Can you work these out from the model? Positions are in its coordinate system, mm. A direction names the side the tool comes from. Round coordinates to 2 decimals unless told otherwise and drop trailing zeros. Write each loop counter-clockwise with the first axis right and the second up, starting at its lowest first coordinate (ties: lowest second). Pieces come first, ordered by that corner, then holes. Notation, with made-up numbers: (-35, 58.5) - (-7, 58.5) arc R7 ccw to (-7, 66.5) - close; hole circle Ø8 at (-23.75, 83.25). An arc over 180 degrees is marked (long way). One line per item, written item: value. Start each with the question number.
(1) I'm going to push flat-ended pins straight in: pin 1 Ø5 at (x, z) = (25.5, 40.5) entering from +Y; pin 2 Ø2 at (x, y) = (36, -7.5) entering from -Z; pin 3 Ø12 at (y, z) = (29, 31.5) entering from +X. Where does each tip first touch, or does it pass through?
(2) I want a section at B-B on x = -19. List the corners of the cut face in (y, z) for me.
(3) If I drill on L1, parallel to X at y = -10, z = 30; L2, parallel to Y at x = 8, z = 18.5; L3, parallel to X at y = -7.85, z = 30, over which ranges is the centre line in solid material (lowest first)? Write a range as from..to.
(4) I want a section at D-D on z = 24. Give the number of separate pieces and of enclosed holes in the cut face, plus the area to 3 significant figures.
(5) I want a section at A-A on y = 18.4. List the corners of the cut face in (x, z) for me, plus the area to 3 significant figures.
(6) I want a section at C-C on y = -7.5. List the corners of the cut face in (x, z) for me.
(7) Thinking about a two-plate mould opening in X: for faces 4 (the face through (9.513, -5.748, 29.58)), 5 (the face through (-4.079, -5.593, 29.58)), 6 (the face through (9.506, 3, 30)), 7 (the face through (-27, -5.6, 20)), which applies, +X half, -X half, draft (parallel to the pull), parting line (faces both ways), or undercut?
(8) On a 3-axis mill with a long thin cutter (end or side, diameter ignored), from which of +Z, -Z, +X, -X, +Y, -Y can I reach the whole of each face in a straight line? I mean faces 1 (the face through (7.985, 8.056, 43.491)), 2 (the face through (-1.228, 35, 30)), 3 (the face through (27, -5.6, 20)). Say none if no direction works.
from build123d import *

# Parameters (mm, degrees)
BOSS_EXTRUDE1_DEPTH      = 60
SKETCH2_R                = 12
SKETCH2_R_2              = 10
BOSS_EXTRUDE3_DEPTH      = 3
SKETCH10_R               = 10
CUT_EXTRUDE3_DEPTH       = 53
SKETCH11_5_R             = 15
CUT_EXTRUDE4_DEPTH       = 23
SKETCH11_R               = 17
SKETCH11_R_2             = 15
BOSS_EXTRUDE7_DEPTH      = 3
BOSS_EXTRUDE7_DEPTH_BACK = 3


with BuildPart() as part:
    # Sketch1 → Boss-Extrude1 (new body)
    with BuildSketch(Plane.XY):
        with BuildLine():
            Line((-47.49441662, -13.6), (52.50558338, -13.6))
            Line((52.50558338, -13.6), (52.50558338, -8.6))
            Line((52.50558338, -8.6), (16.50558338, -8.6))
            ThreePointArc((16.50558338, -8.6), (9.434515568, -5.671067812), (6.50558338, 1.4))
            Line((6.50558338, 1.4), (6.50558338, 41.4))
            Line((6.50558338, 41.4), (-1.227749954, 41.4))
            Line((-1.227749954, 41.4), (-1.227749954, 1.4))
            ThreePointArc((-1.227749954, 1.4), (-4.156682142, -5.671067812), (-11.227749954, -8.6))
            Line((-11.227749954, -8.6), (-47.49441662, -8.6))
            Line((-47.49441662, -8.6), (-47.49441662, -13.6))
        make_face()
    extrude(amount=BOSS_EXTRUDE1_DEPTH)

    # Sketch2 → Boss-Extrude3 (add)
    with BuildSketch(Plane(origin=(0, -8.6, 0), x_dir=(1, 0, 0), z_dir=(0, 1, 0))):
        with Locations((-24.49441662, -30)):
            Circle(SKETCH2_R)
        with Locations((-24.49441662, -30)):
            Circle(SKETCH2_R_2, mode=Mode.SUBTRACT)
        with Locations((29.50558338, -30)):
            Circle(SKETCH2_R)
        with Locations((29.50558338, -30)):
            Circle(SKETCH2_R_2, mode=Mode.SUBTRACT)
    extrude(amount=BOSS_EXTRUDE3_DEPTH)

    # Sketch10 → Cut-Extrude3 (cut)
    with BuildSketch(Plane(origin=(0, -8.6, 0), x_dir=(1, 0, 0), z_dir=(0, 1, 0))):
        with Locations((-24.49441662, -30)):
            Circle(SKETCH10_R)
        with Locations((29.50558338, -30)):
            Circle(SKETCH10_R)
    extrude(amount=-CUT_EXTRUDE3_DEPTH, mode=Mode.SUBTRACT)

    # Sketch11_5 → Cut-Extrude4 (cut)
    with BuildSketch(Plane(origin=(6.50558338, 0, 0), x_dir=(0, 0, -1), z_dir=(1, 0, 0))):
        with Locations((-30, 18.4)):
            Circle(SKETCH11_5_R)
        with BuildLine():
            Line((-60, 41.4), (-60, 31.869694824))
            ThreePointArc((-60, 31.869694824), (-57.186392619, 38.586392619), (-50.469694824, 41.4))
            Line((-50.469694824, 41.4), (-60, 41.4))
        make_face()
        with BuildLine():
            Line((0, 41.4), (-9.606995457, 41.4))
            ThreePointArc((-9.606995457, 41.4), (-3.020943995, 38.379056005), (0, 31.793004543))
            Line((0, 31.793004543), (0, 41.4))
        make_face()
    extrude(amount=-CUT_EXTRUDE4_DEPTH, mode=Mode.SUBTRACT)

    # Sketch11 → Boss-Extrude7 (add, two sides)
    with BuildSketch(Plane(origin=(6.50558338, 0, 0), x_dir=(0, 0, -1), z_dir=(1, 0, 0))) as boss_extrude7_sk:
        with Locations((-30, 18.4)):
            Circle(SKETCH11_R)
        with Locations((-30, 18.4)):
            Circle(SKETCH11_R_2, mode=Mode.SUBTRACT)
    extrude(amount=BOSS_EXTRUDE7_DEPTH)
    extrude(boss_extrude7_sk.sketch, amount=-BOSS_EXTRUDE7_DEPTH_BACK)


solid = part.part
Established:
1. pin 1: y = -5.6
1. pin 2: z = 19.33
1. pin 3: x = 9.51
2. outline: (-13.6, 0) - (-8.6, 0) - (-8.6, 19.33) - (-5.6, 19.33) - (-5.6, 21.64) - (-13.6, 21.64) - close; (-13.6, 38.36) - (-5.6, 38.36) - (-5.6, 40.67) - (-8.6, 40.67) - (-8.6, 60) - (-13.6, 60) - close
3. L1: -47.49..-34.49, -14.49..19.51, 39.51..52.51
3. L2: -13.6..-3.86, 5.88..8.77, 28.03..30.92
3. L3: -36.49..-34.49, -14.49..-12.49, -7.43..12.71, 17.51..19.51, 39.51..41.51
4. separate pieces: 4
4. enclosed holes: 0
4. area: 599 mm2
5. outline: (-1.23, 0) - (6.51, 0) - (6.51, 13) - (9.51, 13) - (9.51, 15) - (-1.23, 15) - close; (-1.23, 45) - (9.51, 45) - (9.51, 47) - (6.51, 47) - (6.51, 60) - (-1.23, 60) - close
5. area: 244 mm2
6. outline: circle Ø24 at (-24.49, 30); (-6.67, 0) - (11.95, 0) - (11.95, 60) - (-6.67, 60) - close; circle Ø24 at (29.51, 30); hole circle Ø20 at (-24.49, 30); hole circle Ø20 at (29.51, 30)
7. face 4: undercut
7. face 5: undercut
7. face 6: +X half
7. face 7: draft
8. face 1: +X
8. face 2: +Z, -Z, -X, +Y
8. face 3: +Z, -Z, +X, +Y
